```python
from build123d import *

# Parameters (mm, degrees)
F0_R          = 5
F1_DEPTH      = 50
F1_DEPTH_BACK = 10
F2_R          = 7.5
F3_DEPTH      = 40
F5_DEPTH      = 10


with BuildPart() as f1:
    # F0 (on Right) → F1 (new body, two sides)
    with BuildSketch(Plane.YZ) as f1_sk:
        Circle(F0_R)
    extrude(amount=F1_DEPTH)
    extrude(f1_sk.sketch, amount=-F1_DEPTH_BACK)

    # F2 (on Right) → F3 (join)
    with BuildSketch(Plane.YZ):
        Circle(F2_R)
    extrude(amount=F3_DEPTH)

    # F4 (on face) → F5 (cut, through all)
    with BuildSketch(Plane(origin=(-10, 0, 0), x_dir=(0, -1, 0), z_dir=(-1, 0, 0))):
        with BuildLine():
            Line((-4, -3), (-4, 3))
            ThreePointArc((-4, 3), (-5, 0), (-4, -3))
        make_face()
        with BuildLine():
            ThreePointArc((4, -3), (5, 0), (4, 3))
            Line((4, 3), (4, -3))
        make_face()
    extrude(amount=-F5_DEPTH, mode=Mode.SUBTRACT)


solid = f1.part
```
Work out the finished part from the listing and answer in its coordinate system (mm). A direction names the side the tool comes from. Give positions to 0.01 mm unless a question says otherwise; leave off trailing zeros. Write each loop counter-clockwise with the first axis right and the second up, starting at its lowest first coordinate (ties: lowest second). Pieces come first, ordered by that corner, then holes.
(1) The part is cut by section A-A on y = 0. Write down the section's boundary in (x, z).
Final values:
outline: (-10, -5) - (0, -5) - (0, -7.5) - (40, -7.5) - (40, -5) - (50, -5) - (50, 5) - (40, 5) - (40, 7.5) - (0, 7.5) - (0, 5) - (-10, 5) - close
(2) The part is cut by section D-D on y = 6. Write down the section's boundary in (x, z).
Final values:
outline: (0, -4.5) - (40, -4.5) - (40, 4.5) - (0, 4.5) - close
(3) Flat-ended cylindrical pins translate along their axes: pin 1 Ø1.5 at (x, y) = (10, -3.5) entering from +Z; pin 2 Ø1.8 at (x, z) = (-2.5, 1.5) entering from +Y; pin 3 Ø1.5 at (y, z) = (-5.5, 3.5) entering from -X. Find the tip coordinate at first contact, or state that the pin passes through.
Final values:
pin 1: stops at z = 6.98
pin 2: stops at y = 4
pin 3: stops at x = 0
(4) Which of the six approach directions +Z, -Z, +X, -X, +Y, -Y give full straight-line access (tool end or side, diameter ignored) to faces 1 (the cylindrical face through (-5, 0, 5)), 2 (the flat face through (40, 2, -5)), 3 (the flat face through (0, 5, 0))?
Final values:
face 1: +Z, -X
face 2: +X
face 3: -X
(5) The part is cut by section C-C on x = 13.5. Write down the section's boundary in (y, z), plus the area to 3 significant figures.
Final values:
outline: circle Ø15 at (0, 0)
area: 177 mm2
(6) Straight lines are drawn through the part: line 1 (X direction, y = 1.75, z = 6.5); line 2 (Y direction, x = -4, z = 2.25). For each, find the intervals that lie inside material, in ascending order.
Final values:
line 1: x = 0 to 40
line 2: y = -4 to 4
(7) The part is cut by section B-B on z = 0. Write down the section's boundary in (x, y), plus the area to 3 significant figures.
Final values:
outline: (-10, -4) - (0, -4) - (0, -7.5) - (40, -7.5) - (40, -5) - (50, -5) - (50, 5) - (40, 5) - (40, 7.5) - (0, 7.5) - (0, 4) - (-10, 4) - close
area: 780 mm2
